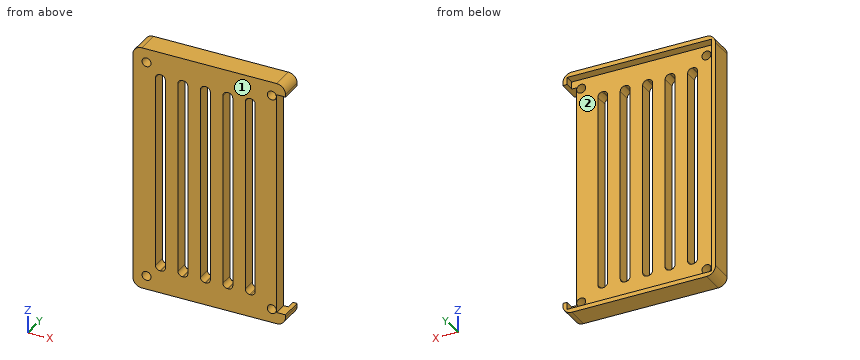
from build123d import *

# Parameters (mm, degrees)
SKETCH_1_W          = 34
SKETCH_1_H          = 55.14
EXTRUDE_1_DEPTH     = 5
SKETCH_2_W          = 32.1
SKETCH_2_H          = 53.24
CUT_EXTRUDE_1_DEPTH = 2
SKETCH_3_W          = 50
SKETCH_3_H          = 10
CUT_EXTRUDE_2_DEPTH = 2
FILLET_3_R          = 2
FILLET_4_R          = 2
FILLET_5_R          = 2
FILLET_6_R          = 2
SKETCH_5_R          = 1
CUT_EXTRUDE_3_DEPTH = 5
CUT_EXTRUDE_5_DEPTH = 5


with BuildPart() as part:
    # 草图1 → 凸台-拉伸1 (new body)
    with BuildSketch(Plane(origin=(0, 0, 0), x_dir=(1, 0, 0), z_dir=(0, 1, 0))):
        with Locations((17, 27.57)):
            Rectangle(SKETCH_1_W, SKETCH_1_H)
    extrude(amount=EXTRUDE_1_DEPTH)

    # 草图2 → 切除-拉伸1 (cut)
    with BuildSketch(Plane(origin=(0, 5, 0), x_dir=(1, 0, 0), z_dir=(0, 1, 0))):
        with Locations((17, 27.57)):
            Rectangle(SKETCH_2_W, SKETCH_2_H)
    extrude(amount=-CUT_EXTRUDE_1_DEPTH, mode=Mode.SUBTRACT)

    # 草图3 → 切除-拉伸2 (cut)
    with BuildSketch(Plane(origin=(34, 0, 0), x_dir=(0, 0, -1), z_dir=(1, 0, 0))):
        with Locations((27.57, 5)):
            Rectangle(SKETCH_3_W, SKETCH_3_H)
    extrude(amount=-CUT_EXTRUDE_2_DEPTH, mode=Mode.SUBTRACT)

    # 圆角3
    fillet_3_edges = [part.edges().sort_by_distance(p)[0] for p in [
        (0, 2.5, 0),
    ]]
    fillet(fillet_3_edges, radius=FILLET_3_R)

    # 圆角4
    fillet_4_edges = [part.edges().sort_by_distance(p)[0] for p in [
        (0, 2.5, -55.14),
    ]]
    fillet(fillet_4_edges, radius=FILLET_4_R)

    # 圆角5
    fillet_5_edges = [part.edges().sort_by_distance(p)[0] for p in [
        (34, 2.5, -55.14),
    ]]
    fillet(fillet_5_edges, radius=FILLET_5_R)

    # 圆角6
    fillet_6_edges = [part.edges().sort_by_distance(p)[0] for p in [
        (34, 2.5, 0),
    ]]
    fillet(fillet_6_edges, radius=FILLET_6_R)

    # 草图5 → 切除-拉伸3 (cut)
    with BuildSketch(Plane(origin=(0, 3, 0), x_dir=(1, 0, 0), z_dir=(0, 1, 0))):
        with Locations(Location((3.05, 52.09, 0), (0, 0, 270))):
            Circle(SKETCH_5_R)
        with Locations(Location((3.05, 3.05, 0), (0, 0, 90))):
            Circle(SKETCH_5_R)
        with Locations(Location((30.95, 3.05, 0), (0, 0, 270))):
            Circle(SKETCH_5_R)
        with Locations(Location((30.95, 52.09, 0), (0, 0, 90))):
            Circle(SKETCH_5_R)
    extrude(amount=-CUT_EXTRUDE_3_DEPTH, mode=Mode.SUBTRACT)

    # 草图6 → 切除-拉伸5 (cut)
    with BuildSketch(Plane(origin=(0, 3, 0), x_dir=(1, 0, 0), z_dir=(0, 1, 0))):
        with BuildLine():
            ThreePointArc((5.05, 49.09), (5.342893219, 49.797106781), (6.05, 50.09))
            Line((6.05, 50.09), (6.254717451, 50.09))
            ThreePointArc((6.254717451, 50.09), (6.961824232, 49.797106781), (7.254717451, 49.09))
            Line((7.254717451, 49.09), (7.254717451, 6.05))
            ThreePointArc((7.254717451, 6.05), (6.961824232, 5.342893219), (6.254717451, 5.05))
            Line((6.254717451, 5.05), (6.05, 5.05))
            ThreePointArc((6.05, 5.05), (5.342893219, 5.342893219), (5.05, 6.05))
            Line((5.05, 6.05), (5.05, 49.09))
        make_face()
        with BuildLine():
            ThreePointArc((10.05, 49.09), (10.342893219, 49.797106781), (11.05, 50.09))
            Line((11.05, 50.09), (11.254717451, 50.09))
            ThreePointArc((11.254717451, 50.09), (11.961824232, 49.797106781), (12.254717451, 49.09))
            Line((12.254717451, 49.09), (12.254717451, 6.05))
            ThreePointArc((12.254717451, 6.05), (11.961824232, 5.342893219), (11.254717451, 5.05))
            Line((11.254717451, 5.05), (11.05, 5.05))
            ThreePointArc((11.05, 5.05), (10.342893219, 5.342893219), (10.05, 6.05))
            Line((10.05, 6.05), (10.05, 49.09))
        make_face()
        with BuildLine():
            ThreePointArc((20.05, 49.09), (20.342893219, 49.797106781), (21.05, 50.09))
            Line((21.05, 50.09), (21.254717451, 50.09))
            ThreePointArc((21.254717451, 50.09), (21.961824232, 49.797106781), (22.254717451, 49.09))
            Line((22.254717451, 49.09), (22.254717451, 6.05))
            ThreePointArc((22.254717451, 6.05), (21.961824232, 5.342893219), (21.254717451, 5.05))
            Line((21.254717451, 5.05), (21.05, 5.05))
            ThreePointArc((21.05, 5.05), (20.342893219, 5.342893219), (20.05, 6.05))
            Line((20.05, 6.05), (20.05, 49.09))
        make_face()
        with BuildLine():
            ThreePointArc((26.05, 5.05), (25.342893219, 5.342893219), (25.05, 6.05))
            Line((25.05, 6.05), (25.05, 49.09))
            ThreePointArc((25.05, 49.09), (25.342893219, 49.797106781), (26.05, 50.09))
            Line((26.05, 50.09), (26.254717451, 50.09))
            ThreePointArc((26.254717451, 50.09), (26.961824232, 49.797106781), (27.254717451, 49.09))
            Line((27.254717451, 49.09), (27.254717451, 6.05))
            ThreePointArc((27.254717451, 6.05), (26.961824232, 5.342893219), (26.254717451, 5.05))
            Line((26.254717451, 5.05), (26.05, 5.05))
        make_face()
        with BuildLine():
            Line((15.05, 49.09), (15.05, 6.05))
            ThreePointArc((15.05, 6.05), (15.342893219, 5.342893219), (16.05, 5.05))
            Line((16.05, 5.05), (16.254717451, 5.05))
            ThreePointArc((16.254717451, 5.05), (16.961824232, 5.342893219), (17.254717451, 6.05))
            Line((17.254717451, 6.05), (17.254717451, 49.09))
            ThreePointArc((17.254717451, 49.09), (16.961824232, 49.797106781), (16.254717451, 50.09))
            Line((16.254717451, 50.09), (16.05, 50.09))
            ThreePointArc((16.05, 50.09), (15.342893219, 49.797106781), (15.05, 49.09))
        make_face()
    extrude(amount=-CUT_EXTRUDE_5_DEPTH, mode=Mode.SUBTRACT)


solid = part.part
Geometry check sheet. Reference: the model listing, model coordinates, mm. Face numbers are marked on the shaded views. Round coordinates to 2 decimals unless told otherwise and drop trailing zeros. Order: outer loops, then holes, each group sorted by start corner. A loop starts at its lowest first (then second) coordinate and runs counter-clockwise, first axis right, second up. Notation, with made-up numbers: (65, 83.25) - (78, 83.25) arc R19 ccw to (78, 120.25) - close; hole circle Ø10 at (35, 82). An arc over 180 degrees is marked (long way). One line per question, with ' | ' between items. Start each with the question number.
(1) Sectioned sample at B-B on x = 30.95. Record the cut outline in (y, z).
(2) Thickness scan on L1, parallel to X at y = 2.3, z = -43; L2, parallel to Z at x = 6, y = 0.3. Record the ranges inside material, lowest first. Write a range as [from, to].
(3) Release check for a two-part mould opening along Z. For the marked faces 1 and 2 record: released by +Z, released by -Z, zero draft, split by the parting line, or undercut.
(4) Sectioned sample at C-C on x = 13.5. Record the cut outline in (y, z).
(5) Sectioned sample at A-A on z = -38. Record the cut outline in (x, y).
(6) Sectioned sample at D-D on y = 3.6. Record the cut outline in (x, z).
(7) Depth check by flat-ended pin: pin 1 Ø12 at (x, z) = (14.5, -20) entering from +Y; pin 2 Ø1.5 at (y, z) = (1.5, -23) entering from +X. Enter the tip coordinate at first touch or a pass-through.
Conclusion:
1) outline: (0, -55.14) - (5, -55.14) - (5, -54.19) - (3, -54.19) - (3, -53.09) - (0, -53.09) - close; (0, -51.09) - (3, -51.09) - (3, -4.05) - (0, -4.05) - close; (0, -2.05) - (3, -2.05) - (3, -0.95) - (5, -0.95) - (5, 0) - (0, 0) - close
2) L1: x = [0, 5.05], [7.25, 10.05], [12.25, 15.05], [17.25, 20.05], [22.25, 25.05], [27.25, 32] | L2: z = [-55.14, -50.09], [-5.05, 0]
3) face 1: zero draft | face 2: undercut
4) outline: (0, -55.14) - (5, -55.14) - (5, -54.19) - (3, -54.19) - (3, -0.95) - (5, -0.95) - (5, 0) - (0, 0) - close
5) outline: (0, 0) - (5.05, 0) - (5.05, 3) - (0.95, 3) - (0.95, 5) - (0, 5) - close; (7.25, 0) - (10.05, 0) - (10.05, 3) - (7.25, 3) - close; (12.25, 0) - (15.05, 0) - (15.05, 3) - (12.25, 3) - close; (17.25, 0) - (20.05, 0) - (20.05, 3) - (17.25, 3) - close; (22.25, 0) - (25.05, 0) - (25.05, 3) - (22.25, 3) - close; (27.25, 0) - (32, 0) - (32, 3) - (27.25, 3) - close
6) outline: (0, -53.14) arc R2 ccw to (2, -55.14) - (32, -55.14) arc R2 ccw to (34, -53.14) - (34, -52.57) - (33.05, -52.57) - (33.05, -54.19) - (0.95, -54.19) - (0.95, -0.95) - (33.05, -0.95) - (33.05, -2.57) - (34, -2.57) - (34, -2) arc R2 ccw to (32, 0) - (2, 0) arc R2 ccw to (0, -2) - close
7) pin 1: stops at y = 3 | pin 2: stops at x = 32
